The model under review builds one solid part; all positions refer to its coordinate system, in mm. A direction names the side the tool comes from. Round coordinates to 2 decimals unless told otherwise and drop trailing zeros. Order: outer loops, then holes, each group sorted by start corner. A loop starts at its lowest first (then second) coordinate and runs counter-clockwise, first axis right, second up. Notation, with made-up numbers: M 69.25,89.25 L 82.25,89.25 A9 ccw 82.25,97.25 Z; hole C 47.5,-40 d7. An arc over 180 degrees is marked long. Answer as a JSON object with one key per item and string values. Group by question number.
1) For faces 1 (the flat face through (123, 265, -2)), 2 (the flat face through (-39, 174.277, 13)), 3 (the flat face through (-37, 299.277, 23)), list the 3-axis set-ups (+Z, -Z, +X, -X, +Y, -Y) from which the entire face can be reached by the end or side of a thin tool; tool diameter is ignored.
2) Consider section B-B, the plane x = 209.5. Write out the cut boundary in (y, z), then the cut area to 3 significant figures.
3) To check wall thickness, follow line 1 (Z direction, x = 115.5, y = 288.5); line 2 (Y direction, x = 144, z = -80.5); line 3 (X direction, y = 267, z = -15). State the ranges of each line that lie inside material, in increasing order.
4) Consider section A-A, the plane z = -87.5. Write out the cut boundary in (x, y).
5) The part is to be moulded in two halves that separate along Y. For faces 4 (the flat face through (54, 329.277, -67)), 5 (the flat face through (-86, 251, -18.057)), 6 (the flat face through (-56, 189.277, 24)), 7 (the flat face through (-106, 234.277, 30)), say which applies: +Y half, -Y half, draft (parallel to the pull), parting line (faces both ways), or undercut.
6) Insertion check: pin 1 Ø1.2 at (x, y) = (121, 207) entering from +Z; pin 2 Ø5.5 at (y, z) = (312, 52.5) entering from +X; pin 3 Ø1 at (x, z) = (83, -113.5) entering from +Y. Each pin has a flat end and moves straight along its axis. Give the tip position at first contact, or say it passes through.
```python
from build123d import *

# Parameters (mm, degrees)
F1_DEPTH  = 123
F2_DEPTH  = 300
F3_R      = 0.5
F4_DEPTH  = 1
F5_W      = 123
F5_H      = 28
F6_DEPTH  = 300
F7_W      = 2.5
F7_H      = 10
F8_DEPTH  = 300
F9_W      = 150
F9_H      = 150
F10_DEPTH = 5
F11_W     = 5
F11_H     = 60
F12_DEPTH = 197.5
F13_W     = 20
F13_H     = 60
F14_DEPTH = 158.5
F15_W     = 20
F15_H     = 60
F15_W_2   = 5
F16_DEPTH = 127.5
F17_W     = 5
F17_H     = 60
F18_DEPTH = 44.5
F19_W     = 5
F19_H     = 60
F20_DEPTH = 1.5
F21_W     = 5
F21_H     = 60
F22_DEPTH = 153.5
F23_W     = 5
F23_H     = 10
F24_DEPTH = 2.5
F25_W     = 5
F25_H     = 10
F26_DEPTH = 2.5
F27_W     = 5
F27_H     = 10
F28_DEPTH = 2.5
F29_W     = 5
F29_H     = 10
F30_DEPTH = 2.5
F31_W     = 5
F31_H     = 10
F32_DEPTH = 2.5
F33_W     = 5
F33_H     = 10
F34_DEPTH = 2.5
F35_W     = 5
F35_H     = 10
F36_DEPTH = 2.5
F37_W     = 5
F37_H     = 10
F38_DEPTH = 2.5
F39_W     = 5
F39_H     = 10
F40_DEPTH = 2.5
F41_W     = 5
F41_H     = 10
F42_DEPTH = 2.5
F43_W     = 5
F43_H     = 10
F44_DEPTH = 2.5
F45_W     = 217.5729006529
F45_H     = 131.9425046444
F46_DEPTH = 5


# Not quite as in the source:
# - a feature names something its author has since deleted; it is built from what else it names


with BuildPart() as f1:
    # F0 (on Right) → F1 (new body)
    with BuildSketch(Plane.YZ):
        Polygon((179.2768240368, 60), (174.2768240368, 60), (174.2768240368, -18.0574953556), (324.2768240368, -18.0574953556), (324.2768240368, -150), (329.2768240368, -150), (329.2768240368, 60), (324.2768240368, 60), (324.2768240368, 0), (314.2768240368, 0), (314.2768240368, 60), (309.2768240368, 60), (309.2768240368, 0), (299.2768240368, 0), (299.2768240368, 60), (294.2768240368, 60), (294.2768240368, 0), (284.2768240368, 0), (284.2768240368, 60), (279.2768240368, 60), (279.2768240368, 0), (269.2768240368, 0), (269.2768240368, 60), (264.2768240368, 60), (264.2768240368, 0), (254.2768240368, 0), (254.2768240368, 60), (249.2768240368, 60), (249.2768240368, 0), (239.2768240368, 0), (239.2768240368, 60), (234.2768240368, 60), (234.2768240368, 0), (224.2768240368, 0), (224.2768240368, 60), (219.2768240368, 60), (219.2768240368, 0), (209.2768240368, 0), (209.2768240368, 60), (204.2768240368, 60), (204.2768240368, 0), (194.2768240368, 0), (194.2768240368, 60), (189.2768240368, 60), (189.2768240368, 0), (179.2768240368, 0), align=None)
    extrude(amount=F1_DEPTH)

    # F0 (on Right) → F2 (join)
    with BuildSketch(Plane.YZ):
        Polygon((179.2768240368, 60), (174.2768240368, 60), (174.2768240368, -18.0574953556), (324.2768240368, -18.0574953556), (324.2768240368, -150), (329.2768240368, -150), (329.2768240368, 60), (324.2768240368, 60), (324.2768240368, 0), (314.2768240368, 0), (314.2768240368, 60), (309.2768240368, 60), (309.2768240368, 0), (299.2768240368, 0), (299.2768240368, 60), (294.2768240368, 60), (294.2768240368, 0), (284.2768240368, 0), (284.2768240368, 60), (279.2768240368, 60), (279.2768240368, 0), (269.2768240368, 0), (269.2768240368, 60), (264.2768240368, 60), (264.2768240368, 0), (254.2768240368, 0), (254.2768240368, 60), (249.2768240368, 60), (249.2768240368, 0), (239.2768240368, 0), (239.2768240368, 60), (234.2768240368, 60), (234.2768240368, 0), (224.2768240368, 0), (224.2768240368, 60), (219.2768240368, 60), (219.2768240368, 0), (209.2768240368, 0), (209.2768240368, 60), (204.2768240368, 60), (204.2768240368, 0), (194.2768240368, 0), (194.2768240368, 60), (189.2768240368, 60), (189.2768240368, 0), (179.2768240368, 0), align=None)
    extrude(amount=-F2_DEPTH)

    # F3 (on face) → F4, piece 2 (join)
    with BuildSketch(Plane(origin=(0, 329.2768240368, 0), x_dir=(-1, 0, 0), z_dir=(0, 1, 0))):
        with Locations((-82.5385674834, -48.5965646803)):
            Circle(F3_R)
        with Locations((31.1017241329, -28.6999493837)):
            Circle(F3_R)
    extrude(amount=F4_DEPTH)

    # F5 (on face) → F6 (cut)
    with BuildSketch(Plane(origin=(0, 329.2768240368, 0), x_dir=(-1, 0, 0), z_dir=(0, 1, 0))):
        with Locations((-61.5, 46)):
            Rectangle(F5_W, F5_H)
    extrude(amount=-F6_DEPTH, mode=Mode.SUBTRACT)

    # F7 (on face) → F8 (cut)
    with BuildSketch(Plane(origin=(0, 329.2768240368, 0), x_dir=(-1, 0, 0), z_dir=(0, 1, 0))):
        with Locations((-1.25, 27)):
            Rectangle(F7_W, F7_H)
        with Locations((1.25, 55)):
            Rectangle(F7_W, F7_H)
        with Locations((-121.75, 27)):
            Rectangle(F7_W, F7_H)
    extrude(amount=-F8_DEPTH, mode=Mode.SUBTRACT)



with BuildPart() as f4:
    # F3 (on face) → F4 (new body)
    with BuildSketch(Plane(origin=(0, 329.2768240368, 0), x_dir=(-1, 0, 0), z_dir=(0, 1, 0))):
        with Locations((-203.3374607563, -30)):
            Circle(F3_R)
    extrude(amount=F4_DEPTH)


with BuildPart() as f1_1:
    add(f1.part)

    add(f4.part)  # F10 merges F4
    # F9 (on face) → F10 (join)
    with BuildSketch(Plane(origin=(0, 329.2768240368, 0), x_dir=(-1, 0, 0), z_dir=(0, 1, 0))):
        with Locations((-198, -75)):
            Rectangle(F9_W, F9_H)
    extrude(amount=-F10_DEPTH)

    # F11 (on face) → F12 (cut)
    with BuildSketch(Plane(origin=(-300, 0, 0), x_dir=(0, -1, 0), z_dir=(-1, 0, 0))):
        with Locations((-326.7768240368, 30)):
            Rectangle(F11_W, F11_H)
        with Locations((-311.7768240368, 30)):
            Rectangle(F11_W, F11_H)
    extrude(amount=-F12_DEPTH, mode=Mode.SUBTRACT)

    # F13 (on face) → F14 (cut)
    with BuildSketch(Plane(origin=(-300, 0, 0), x_dir=(0, -1, 0), z_dir=(-1, 0, 0))):
        with Locations((-289.2768240368, 30)):
            Rectangle(F13_W, F13_H)
    extrude(amount=-F14_DEPTH, mode=Mode.SUBTRACT)

    # F15 (on face) → F16 (cut)
    with BuildSketch(Plane(origin=(-300, 0, 0), x_dir=(0, -1, 0), z_dir=(-1, 0, 0))):
        with Locations((-259.2768240368, 30)):
            Rectangle(F15_W, F15_H)
        with Locations((-191.7768240368, 30)):
            Rectangle(F15_W_2, F15_H)
    extrude(amount=-F16_DEPTH, mode=Mode.SUBTRACT)

    # F17 (on face) → F18 (cut)
    with BuildSketch(Plane(origin=(-300, 0, 0), x_dir=(0, -1, 0), z_dir=(-1, 0, 0))):
        with Locations((-236.7768240368, 30)):
            Rectangle(F17_W, F17_H)
        with Locations((-206.7768240368, 30)):
            Rectangle(F17_W, F17_H)
    extrude(amount=-F18_DEPTH, mode=Mode.SUBTRACT)

    # F19 (on face) → F20 (cut)
    with BuildSketch(Plane(origin=(-300, 0, 0), x_dir=(0, -1, 0), z_dir=(-1, 0, 0))):
        with Locations((-221.7768240368, 30)):
            Rectangle(F19_W, F19_H)
    extrude(amount=-F20_DEPTH, mode=Mode.SUBTRACT)

    # F21 (on face) → F22 (cut)
    with BuildSketch(Plane(origin=(-300, 0, 0), x_dir=(0, -1, 0), z_dir=(-1, 0, 0))):
        with Locations((-176.7768240368, 30)):
            Rectangle(F21_W, F21_H)
    extrude(amount=-F22_DEPTH, mode=Mode.SUBTRACT)

    # F23 (on face) → F24 (cut)
    with BuildSketch(Plane(origin=(-298.5, 0, 0), x_dir=(0, -1, 0), z_dir=(-1, 0, 0))):
        with Locations((-221.7768240368, 55)):
            Rectangle(F23_W, F23_H)
    extrude(amount=-F24_DEPTH, mode=Mode.SUBTRACT)

    # F25 (on face) → F26 (cut)
    with BuildSketch(Plane(origin=(-255.5, 0, 0), x_dir=(0, -1, 0), z_dir=(-1, 0, 0))):
        with Locations((-236.7768240368, 55)):
            Rectangle(F25_W, F25_H)
    extrude(amount=-F26_DEPTH, mode=Mode.SUBTRACT)

    # F27 (on face) → F28 (cut)
    with BuildSketch(Plane(origin=(-255.5, 0, 0), x_dir=(0, -1, 0), z_dir=(-1, 0, 0))):
        with Locations((-206.7768240368, 55)):
            Rectangle(F27_W, F27_H)
    extrude(amount=-F28_DEPTH, mode=Mode.SUBTRACT)

    # F29 (on face) → F30 (cut)
    with BuildSketch(Plane(origin=(-172.5, 0, 0), x_dir=(0, -1, 0), z_dir=(-1, 0, 0))):
        with Locations((-251.7768240368, 55)):
            Rectangle(F29_W, F29_H)
    extrude(amount=-F30_DEPTH, mode=Mode.SUBTRACT)

    # F31 (on face) → F32 (cut)
    with BuildSketch(Plane(origin=(-172.5, 0, 0), x_dir=(0, -1, 0), z_dir=(-1, 0, 0))):
        with Locations((-191.7768240368, 55)):
            Rectangle(F31_W, F31_H)
    extrude(amount=-F32_DEPTH, mode=Mode.SUBTRACT)

    # F33 (on face) → F34 (cut)
    with BuildSketch(Plane(origin=(-172.5, 0, 0), x_dir=(0, -1, 0), z_dir=(-1, 0, 0))):
        with Locations((-266.7768240368, 55)):
            Rectangle(F33_W, F33_H)
    extrude(amount=-F34_DEPTH, mode=Mode.SUBTRACT)

    # F35 (on face) → F36 (cut)
    with BuildSketch(Plane(origin=(-146.5, 0, 0), x_dir=(0, -1, 0), z_dir=(-1, 0, 0))):
        with Locations((-176.7768240368, 55)):
            Rectangle(F35_W, F35_H)
    extrude(amount=-F36_DEPTH, mode=Mode.SUBTRACT)

    # F37 (on face) → F38 (cut)
    with BuildSketch(Plane(origin=(-141.5, 0, 0), x_dir=(0, -1, 0), z_dir=(-1, 0, 0))):
        with Locations((-281.7768240368, 55)):
            Rectangle(F37_W, F37_H)
    extrude(amount=-F38_DEPTH, mode=Mode.SUBTRACT)

    # F39 (on face) → F40 (cut)
    with BuildSketch(Plane(origin=(-141.5, 0, 0), x_dir=(0, -1, 0), z_dir=(-1, 0, 0))):
        with Locations((-296.7768240368, 55)):
            Rectangle(F39_W, F39_H)
    extrude(amount=-F40_DEPTH, mode=Mode.SUBTRACT)

    # F41 (on face) → F42 (join)
    with BuildSketch(Plane(origin=(-102.5, 0, 0), x_dir=(0, -1, 0), z_dir=(-1, 0, 0))):
        with Locations((-311.7768240368, 55)):
            Rectangle(F41_W, F41_H)
    extrude(amount=F42_DEPTH)

    # F43 (on face) → F44 (cut)
    with BuildSketch(Plane(origin=(-102.5, 0, 0), x_dir=(0, -1, 0), z_dir=(-1, 0, 0))):
        with Locations((-326.7768240368, 55)):
            Rectangle(F43_W, F43_H)
    extrude(amount=-F44_DEPTH, mode=Mode.SUBTRACT)

    # F45 (on face) → F46 (cut)
    with BuildSketch(Plane(origin=(0, 329.2768240368, 0), x_dir=(-1, 0, 0), z_dir=(0, 1, 0))):
        with Locations((191.2135496736, -84.0287476778)):
            Rectangle(F45_W, F45_H)
    extrude(amount=-F46_DEPTH, mode=Mode.SUBTRACT)


solid = f1_1.part
```
Results list:
{
 "1": {"face 1": "+Z, -Z, +X, -Y", "face 2": "+Z, -Z, +X, -X, -Y", "face 3": "+Z, +X, -X"},
 "2": {"outline": "M 324.28,-150 L 329.28,-150 L 329.28,0 L 324.28,0 Z", "area": "750 mm^2"},
 "3": {"line 1": "-18.06 to 0", "line 2": "324.28 to 329.28", "line 3": "-300 to 123"},
 "4": {"outline": "M -82.43,324.28 L 273,324.28 L 273,329.28 L -82.43,329.28 Z"},
 "5": {"face 4": "+Y half", "face 5": "draft", "face 6": "undercut", "face 7": "undercut"},
 "6": {"pin 1": "z = 32", "pin 2": "x = 0", "pin 3": "y = 329.28"}
}
